Here's how the part is built. I have some questions about the finished solid (model axes, mm). Give positions to 0.01 mm unless a question says otherwise; leave off trailing zeros. Loops run counter-clockwise (first coordinate to the right, second up) from the corner with the lowest first, then second, coordinate; pieces in that order, holes last.
Q1. Will these pins go through, and if not, where does the flat tip stop? P1, Ø1.4, axis at x = 1, y = 2.5, coming from the +Z side; P2, Ø0.5, axis at x = 1.5, y = -2.5, coming from the -Z side; P3, Ø1, axis at x = 1.5, z = 75, coming from the +Y side.
Q2. If we section it at B-B (x = 2.3): Give the number of separate pieces and of enclosed holes in the cut face, plus the area to 3 significant figures.
Q3. If we section it at A-A (z = -18): Please give me the cut outline in (x, y).
Q4. I need wall thicknesses on line 1 (Y direction, x = 1.3, z = -6.2); line 2 (Y direction, x = 2.5, z = 0); line 3 (Z direction, x = 1.6, y = -2.5). Which ranges of each line are inside material? Lowest first, please.
from build123d import *

# Parameters (mm, degrees)
SKETCH1_W           = 152.4
SKETCH1_H           = 146.04
BOSS_EXTRUDE1_DEPTH = 3.18
SKETCH3_R           = 1.4
SKETCH3_W           = 10
SKETCH3_H           = 3.18
BOSS_EXTRUDE5_DEPTH = 3.18
CUT_EXTRUDE2_DEPTH  = 4.18
CUT_EXTRUDE3_DEPTH  = 4.18
SKETCH6_R           = 1.6
CUT_EXTRUDE6_DEPTH  = 4.18


with BuildPart() as part:
    # Sketch1 → Boss-Extrude1 (new body)
    with BuildSketch(Plane(origin=(0, 0, 0), x_dir=(0, 0, -1), z_dir=(1, 0, 0))):
        Rectangle(SKETCH1_W, SKETCH1_H)
    extrude(amount=BOSS_EXTRUDE1_DEPTH)

    # Sketch3 → Boss-Extrude5 (add)
    with BuildSketch(Plane.ZY):
        Polygon((0, 73.02), (5, 73.02), (5, 76.2), (-5, 76.2), (-5, 73.02), align=None)
        with Locations((0, 74.61)):
            Circle(SKETCH3_R, mode=Mode.SUBTRACT)
        with Locations((0, -74.61)):
            Rectangle(SKETCH3_W, SKETCH3_H)
        with Locations((0, -74.61)):
            Circle(SKETCH3_R, mode=Mode.SUBTRACT)
    extrude(amount=-BOSS_EXTRUDE5_DEPTH)

    # Sketch4 → Cut-Extrude2 (cut, through all)
    with BuildSketch(Plane(origin=(0, 0, 0), x_dir=(0, 0, -1), z_dir=(1, 0, 0))):
        Polygon((-76.2, -5), (-76.2, 5), (-73.02, 5), (-73.02, 1.47), (-70.02, 1.47), (-70.02, 3.25), (-67.42, 3.25), (-67.42, 1.47), (-63.2, 1.47), (-63.2, -1.47), (-67.42, -1.47), (-67.42, -3.25), (-70.02, -3.25), (-70.02, -1.47), (-73.02, -1.47), (-73.02, -5), align=None)
    extrude(amount=CUT_EXTRUDE2_DEPTH, mode=Mode.SUBTRACT)

    # Sketch5 → Cut-Extrude3 (cut, through all)
    with BuildSketch(Plane.ZY):
        Polygon((-70.02, -1.47), (-73.02, -1.47), (-73.02, -5), (-76.2, -5), (-76.2, 5), (-73.02, 5), (-73.02, 1.47), (-70.02, 1.47), (-70.02, 3.25), (-67.42, 3.25), (-67.42, 1.47), (-63.2, 1.47), (-63.2, -1.47), (-67.42, -1.47), (-67.42, -3.25), (-70.02, -3.25), align=None)
    extrude(amount=-CUT_EXTRUDE3_DEPTH, mode=Mode.SUBTRACT)

    # Sketch6 → Cut-Extrude6 (cut, through all)
    with BuildSketch(Plane.ZY):
        with Locations((46.2, -58.02)):
            Circle(SKETCH6_R)
        with Locations((44.6, -9.72)):
            Circle(SKETCH6_R)
        with Locations((-6.2, -52.92)):
            Circle(SKETCH6_R)
        with Locations((-6.2, -25.02)):
            Circle(SKETCH6_R)
    extrude(amount=-CUT_EXTRUDE6_DEPTH, mode=Mode.SUBTRACT)


solid = part.part
Check sheet entries:
1. P1: stops at z = 73.02
1. P2: stops at z = -73.02
1. P3: stops at y = 73.02
2. separate pieces: 1
2. enclosed holes: 6
2. area: 22,100 mm2
3. outline: (0, -73.02) - (3.18, -73.02) - (3.18, 73.02) - (0, 73.02) - close
4. line 1: y = -73.02 to -54.52, -51.32 to -26.62, -23.42 to 73.02
4. line 2: y = -76.2 to -76.01, -73.21 to 73.21, 76.01 to 76.2
4. line 3: z = -73.02 to -70.02, -67.42 to 67.42, 70.02 to 73.02
